```python
from build123d import *

# Parameters (mm, degrees)
SKETCH2_R           = 3.2639
BOSS_EXTRUDE1_DEPTH = 1.5875
FILLET1_R           = 2.54


with BuildPart() as part:
    # Sketch2 → Boss-Extrude1 (new body)
    with BuildSketch(Plane(origin=(0, 55.360225049, -4.608794225), x_dir=(-1, 0, 0), z_dir=(1.3350431871117514e-14, -0.9965525450230818, 0.0829639982644206))):
        Polygon((255.547712488, -35.085636701), (314.736370081, -108.545763081), (319.072942794, -88.62551032), (275.934530116, -35.085636701), align=None)
        with Locations(Location((291.32288887, -66.835636701, 0), (0, 0, 270))):
            Circle(SKETCH2_R, mode=Mode.SUBTRACT)
    extrude(amount=BOSS_EXTRUDE1_DEPTH)

    # Fillet1
    fillet1_edges = [part.edges().sort_by_distance(p)[0] for p in [
        (-275.934530116, 57.480056169, 30.421738996),
        (-319.072942794, 61.921938151, 83.777036311),
        (-314.736370081, 63.574601966, 103.628614898),
        (-255.547712488, 57.480056169, 30.421738996),
    ]]
    fillet(fillet1_edges, radius=FILLET1_R)


solid = part.part
```
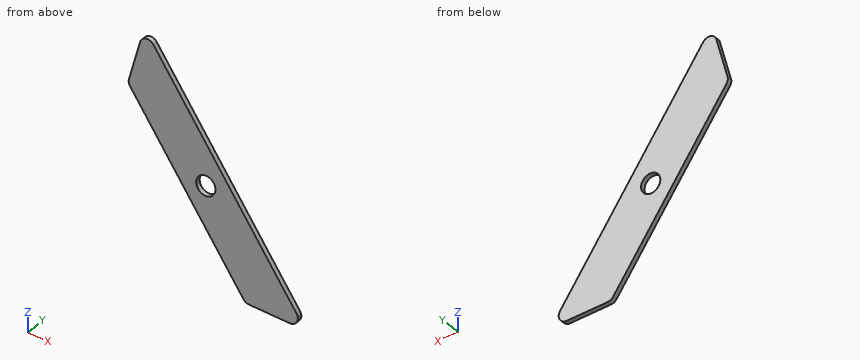
Here's how the part is built. I have some questions about the finished solid (model axes, mm). Coordinates: 2 decimals unless noted, no trailing zeros. Order: outer loops, then holes, each group sorted by start corner. A loop starts at its lowest first (then second) coordinate and runs counter-clockwise, first axis right, second up. Notation, with made-up numbers: (88, -4) -> (100, -4) arc R32 cw to (100, 32) -> close; hole circle Ø9 at (77.25, 43.25). An arc over 180 degrees is marked (long way). Return JSON: item names as keys, results as strings.
1) If we section it at A-A on z = 74: List the corners of the cut face in (x, y) for me, plus the area to 3 significant figures.
Conclusion:
{"outline": "(-311.22, 61.9) -> (-311.11, 60.31) -> (-290.73, 60.31) -> (-290.83, 61.9) -> close", "area": "32.5 mm²"}
2) If we section it at B-B on x = -265.5: List the corners of the cut face in (y, z) for me.
Conclusion:
{"outline": "(56.69, 30.49) -> (58.27, 30.36) -> (59.3, 42.67) -> (57.71, 42.8) -> close"}
3) I'm going to push flat-ended pins straight in: P1, Ø1.5, axis at y = 60, z = 48, coming from the -X side; P2, Ø4, axis at x = -282, y = 58.5, coming from the +Z side. Where does each tip first touch, or does it pass through?
Conclusion:
{"P1": "stops at x = -290.78", "P2": "stops at z = 65.28"}
4) If I drill on probe 1 along Z at (x, y) = (-292, 59.25); probe 2 along X at (y, z) = (60.25, 61); probe 3 along Y at (x, z) = (-294.5, 78), over which ranges is the centre line in solid material (lowest first)?
Conclusion:
{"probe 1": "z = 50.28 to 58.93", "probe 2": "x = -300.67 to -294.41, -288.23 to -280.29", "probe 3": "y = 60.64 to 62.24"}
